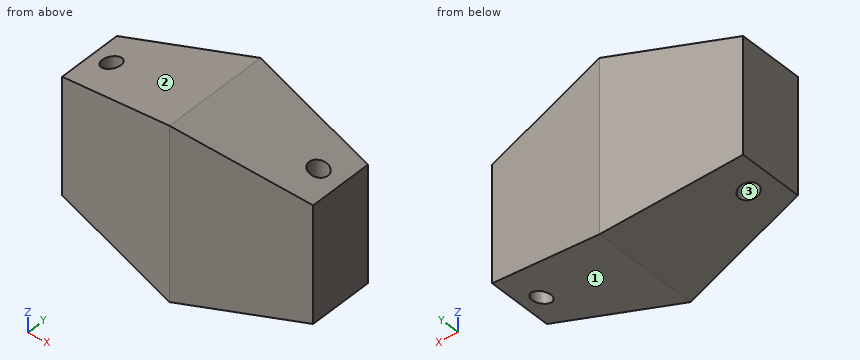
```python
from build123d import *

# Parameters (mm, degrees)
SKETCH1_W               = 80
SKETCH1_H               = 35
BOSS_EXTRUDE1_DEPTH     = 55
CUT_EXTRUDE1_DEPTH      = 55
CUT_EXTRUDE2_DEPTH      = 71.222859526
CUT_EXTRUDE2_DEPTH_BACK = 71.222859526
CUT_EXTRUDE3_DEPTH      = 71.222859526
CUT_EXTRUDE3_DEPTH_BACK = 71.222859526
SKETCH6_R               = 3


with BuildPart() as part:
    # Sketch1 → Boss-Extrude1 (new body)
    with BuildSketch(Plane.XY):
        Rectangle(SKETCH1_W, SKETCH1_H)
    extrude(amount=BOSS_EXTRUDE1_DEPTH)

    # Sketch2 → Cut-Extrude1 (cut)
    with BuildSketch(Plane(origin=(0, 17.5, 0), x_dir=(1, 0, 0), z_dir=(0, 1, 0))):
        Polygon((-40, -55), (0, -55), (-40, -46), align=None)
        Polygon((40, -46), (0, -55), (40, -55), align=None)
        Polygon((0, 0), (40, -9), (40, 0), align=None)
        Polygon((-40, 0), (-40, -9), (0, 0), align=None)
    extrude(amount=-CUT_EXTRUDE1_DEPTH, mode=Mode.SUBTRACT)

    # Sketch5 → Cut-Extrude2 (cut, two sides: drawn at the far end of the back side and taken through both)
    with BuildSketch(Plane.XY.offset(-CUT_EXTRUDE2_DEPTH_BACK)):
        Polygon((40, 17.5), (40, 10.5), (0, 17.5), align=None)
        Polygon((-40, 17.5), (0, 17.5), (-40, 10.5), align=None)
        Polygon((40, -17.5), (0, -17.5), (40, -10.5), align=None)
        Polygon((-40, -10.5), (-40, -17.5), (0, -17.5), align=None)
    extrude(amount=CUT_EXTRUDE2_DEPTH + CUT_EXTRUDE2_DEPTH_BACK, mode=Mode.SUBTRACT)

    # Sketch6 → Cut-Extrude3 (cut, two sides: drawn at the far end of the back side and taken through both)
    with BuildSketch(Plane.XY.offset(-CUT_EXTRUDE3_DEPTH_BACK)):
        with Locations((-33, 0)):
            Circle(SKETCH6_R)
        with Locations((33, 0)):
            Circle(SKETCH6_R)
    extrude(amount=CUT_EXTRUDE3_DEPTH + CUT_EXTRUDE3_DEPTH_BACK, mode=Mode.SUBTRACT)


solid = part.part
```
The listing builds one solid part. Answer for the finished solid, in the listing's coordinates (mm). Face numbers are marked on the shaded views. Round coordinates to 2 decimals unless told otherwise and drop trailing zeros. Order: outer loops, then holes, each group sorted by start corner. A loop starts at its lowest first (then second) coordinate and runs counter-clockwise, first axis right, second up. Notation, with made-up numbers: (0.5, -40) -> (10.5, -40) arc R7 cw to (10.5, -33) -> close; hole circle Ø9 at (-28.5, 16). An arc over 180 degrees is marked (long way). Answer as CSV lines item,"result". Start each with the question number.
(1) The part is cut by section A-A (y = 0). Determine the outline of the cut face in (x, z).
(2) The part is cut by section D-D (y = 8). Determine the outline of the cut face in (x, z).
(3) Find the intervals of material crossed by probe 1 along X at (y, z) = (0, 22); probe 2 along Y at (x, z) = (-33, 9) (3 decimals); probe 3 along Z at (x, y) = (4, 0), in increasing order. Write a range as from..to.
(4) The part is cut by section B-B (z = 33.5). Determine the outline of the cut face in (x, y).
(5) The part is cut by section C-C (x = -33). Determine the outline of the cut face in (y, z) (3 decimals).
(6) For a pull along X with two mould halves and no side action, classify the marked faces 1, 2 and 3 as +X half, -X half, draft (parallel to the pull), parting line (faces both ways), or undercut.
(7) Flat-ended cylindrical pins translate along their axes: pin 1 Ø10 at (x, y) = (-27.5, 12.5) entering from -Z; pin 2 Ø7 at (x, y) = (33, 0) entering from +Z; pin 3 Ø7 at (x, y) = (-33, 0) entering from -Z. Find the tip coordinate at first contact, or state that the pin passes through.
Evaluation:
1,outline,"(-40, 9) -> (-36, 8.1) -> (-36, 46.9) -> (-40, 46) -> close; (-30, 6.75) -> (0, 0) -> (30, 6.75) -> (30, 48.25) -> (0, 55) -> (-30, 48.25) -> close; (36, 8.1) -> (40, 9) -> (40, 46) -> (36, 46.9) -> close"
2,outline,"(-40, 9) -> (0, 0) -> (40, 9) -> (40, 46) -> (0, 55) -> (-40, 46) -> close"
3,probe 1,"-40..-36, -30..30, 36..40"
3,probe 2,"-11.725..-3, 3..11.725"
3,probe 3,"0.9..54.1"
4,outline,"(-40, -10.5) -> (0, -17.5) -> (40, -10.5) -> (40, 10.5) -> (0, 17.5) -> (-40, 10.5) -> close; hole circle Ø6 at (-33, 0); hole circle Ø6 at (33, 0)"
5,outline,"(-11.725, 7.425) -> (-3, 7.425) -> (-3, 47.575) -> (-11.725, 47.575) -> close; (3, 7.425) -> (11.725, 7.425) -> (11.725, 47.575) -> (3, 47.575) -> close"
6,face 1,"+X half"
6,face 2,"-X half"
6,face 3,"undercut"
7,pin 1,"z = 5.06"
7,pin 2,"z = 48.36"
7,pin 3,"z = 6.64"
